Read the model definition and answer for the solid it produces. Units are mm, in the model's axes. A direction names the side the tool comes from. Coordinates: 2 decimals unless noted, no trailing zeros. Write each loop counter-clockwise with the first axis right and the second up, starting at its lowest first coordinate (ties: lowest second). Pieces come first, ordered by that corner, then holes. Notation, with made-up numbers: (23, 88) -> (45, 88) arc R14 cw to (45, 92) -> close; hole circle Ø1 at (75, 53). An arc over 180 degrees is marked (long way). Write item = value, one per line. Start each with the question number.
1) Find the intervals of material crossed by line 1 along X through (y, z) = (0.9, -17.5); line 2 along Z through (x, y) = (-32, 1.05); line 3 along Z through (x, y) = (-3, -0.95), in increasing order. Write a range as from..to.
2) Section A-A (y = -0.9) is taken. Count the separate pieces of the cut face and the enclosed holes in it, plus the area to 3 significant figures.
3) Section B-B (x = 0) is taken. Determine the outline of the cut face in (y, z).
4) A tool of negligible diameter and unlimited length cuts with its end or side. For faces 1 (the face through (0, 0, 0)), 2 (the face through (-16, -1, -18)), 3 (the face through (16, -1, 18)), from which of +Z, -Z, +X, -X, +Y, -Y can it reach the whole face along a straight path? Write none if from no direction.
5) Section C-C (z = -14) is taken. Determine the outline of the cut face in (x, y), plus the area to 3 significant figures.
6) For a pull along X with two mould halves and no side action, classify faces 4 (the face through (-34.4, 0.99, -19.43)), 5 (the face through (-16, -1, 18)), 6 (the face through (33, -1, 0)) as released by +X, released by -X, zero draft, split by the parting line, or undercut.
7) Flat-ended cylindrical pins translate along their axes: pin 1 Ø1 at (x, y) = (10.5, -1.5) entering from +Z; pin 2 Ø1.6 at (x, y) = (-10.5, -1) entering from -Z; pin 3 Ø4 at (x, z) = (32, 17.5) entering from +Y; pin 4 Ø1 at (x, z) = (-4.5, -14) entering from -Y. Find the tip coordinate at first contact, or state that the pin passes through.
from build123d import *

# Parameters (mm, degrees)
BOSS_EXTRUDE1_DEPTH = 2
BOSS_EXTRUDE2_DEPTH = 2
SKETCH3_R           = 1.75
CUT_EXTRUDE1_DEPTH  = 10


with BuildPart() as part:
    # Sketch1 → Boss-Extrude1 (new body)
    with BuildSketch(Plane(origin=(0, 0, 0), x_dir=(1, 0, 0), z_dir=(0, 1, 0))):
        with BuildLine():
            Line((-33, -20), (33, -20))
            ThreePointArc((33, -20), (34.414213562, -19.414213562), (35, -18))
            Line((35, -18), (35, 18))
            ThreePointArc((35, 18), (34.414213562, 19.414213562), (33, 20))
            Line((33, 20), (-33, 20))
            ThreePointArc((-33, 20), (-34.414213562, 19.414213562), (-35, 18))
            Line((-35, 18), (-35, -18))
            ThreePointArc((-35, -18), (-34.414213562, -19.414213562), (-33, -20))
        make_face()
    extrude(amount=BOSS_EXTRUDE1_DEPTH)

    # Sketch2 → Boss-Extrude2 (add)
    with BuildSketch(Plane.XZ):
        with BuildLine():
            Line((-32, 18), (32, 18))
            ThreePointArc((32, 18), (33.414213562, 17.414213562), (34, 16))
            Line((34, 16), (34, -16))
            ThreePointArc((34, -16), (33.414213562, -17.414213562), (32, -18))
            Line((32, -18), (-32, -18))
            ThreePointArc((-32, -18), (-33.414213562, -17.414213562), (-34, -16))
            Line((-34, -16), (-34, 16))
            ThreePointArc((-34, 16), (-33.414213562, 17.414213562), (-32, 18))
        make_face()
        with BuildLine():
            Line((-31, 17), (31, 17))
            ThreePointArc((31, 17), (32.414213562, 16.414213562), (33, 15))
            Line((33, 15), (33, -15))
            ThreePointArc((33, -15), (32.414213562, -16.414213562), (31, -17))
            Line((31, -17), (-31, -17))
            ThreePointArc((-31, -17), (-32.414213562, -16.414213562), (-33, -15))
            Line((-33, -15), (-33, 15))
            ThreePointArc((-33, 15), (-32.414213562, 16.414213562), (-31, 17))
        make_face(mode=Mode.SUBTRACT)
    extrude(amount=BOSS_EXTRUDE2_DEPTH)

    # Sketch3 → Cut-Extrude1 (cut)
    with BuildSketch(Plane(origin=(0, 2, 0), x_dir=(1, 0, 0), z_dir=(0, 1, 0))):
        with Locations(Location((-32, 17.5, 0), (0, 0, 270))):
            Circle(SKETCH3_R)
        with Locations(Location((0, 17.5, 0), (0, 0, 270))):
            Circle(SKETCH3_R)
        with Locations(Location((32, 17.5, 0), (0, 0, 270))):
            Circle(SKETCH3_R)
        with Locations(Location((32, -17.5, 0), (0, 0, 270))):
            Circle(SKETCH3_R)
        with Locations(Location((0, -17.5, 0), (0, 0, 270))):
            Circle(SKETCH3_R)
        with Locations(Location((-32, -17.5, 0), (0, 0, 270))):
            Circle(SKETCH3_R)
    extrude(amount=-CUT_EXTRUDE1_DEPTH, mode=Mode.SUBTRACT)


solid = part.part
Answer key:
q1.line_1 = -35..-33.75, -30.25..-1.75, 1.75..30.25, 33.75..35
q1.line_2 = -20..-19.25, -15.75..15.75, 19.25..20
q1.line_3 = -18..-17, 17..18
q2.separate_pieces = 6
q2.enclosed_holes = 0
q2.area = 181 mm^2
q3.outline = (0, -20) -> (2, -20) -> (2, -19.25) -> (0, -19.25) -> close; (0, -15.75) -> (2, -15.75) -> (2, 15.75) -> (0, 15.75) -> close; (0, 19.25) -> (2, 19.25) -> (2, 20) -> (0, 20) -> close
q4.face_1 = -Y
q4.face_2 = -Z, +X, -X, -Y
q4.face_3 = +Z, +X, -X, -Y
q5.outline = (-35, 0) -> (-34, 0) -> (-34, -2) -> (-33, -2) -> (-33, 0) -> (33, 0) -> (33, -2) -> (34, -2) -> (34, 0) -> (35, 0) -> (35, 2) -> (-35, 2) -> close
q5.area = 144 mm^2
q6.face_4 = released by -X
q6.face_5 = zero draft
q6.face_6 = undercut
q7.pin_1 = 18
q7.pin_2 = -18
q7.pin_3 = 2
q7.pin_4 = 0
